Part model, mm, in its own coordinate system. Face numbers are marked on the shaded views. A direction names the side the tool comes from. Coordinates: 2 decimals unless noted, no trailing zeros. Loops run counter-clockwise (first coordinate to the right, second up) from the corner with the lowest first, then second, coordinate; pieces in that order, holes last. Notation, with made-up numbers: (65, 5.25) -> (110, 5.25) arc R26 ccw to (110, 38.25) -> close; hole circle Ø11 at (86.5, 69). An arc over 180 degrees is marked (long way). Use one line per item in the form item = value. Start each with the question number.
(1) 3-axis set-ups, long thin cutter, end or side, ignore diameter. For the marked faces 1 and 2: which of +Z, -Z, +X, -X, +Y, -Y reach the whole face in a straight line?
(2) Band-saw the part on D-D on x = -31. Give the cut face in (y, z), then the cut area to 3 significant figures.
(3) Band-saw the part on B-B on x = 0. Give the cut face in (y, z), then the cut area to 3 significant figures.
(4) Pin check, flat tips, straight feed: P1, Ø6, axis at x = 22, y = 15, coming from the -Z side; P2, Ø1.5, axis at x = 22.5, y = 5.5, coming from the -Z side; P3, Ø2, axis at x = -4, y = 7, coming from the -Z side. Stop position of each tip, or through.
(5) Mould opens along X. For the marked faces 3, 4 and 5 say: +X half, -X half, draft (parallel to the pull), parting line (faces both ways), or undercut.
(6) Band-saw the part on C-C on y = 31.5. Give the cut face in (x, z), then the cut area to 3 significant figures.
(7) Drill centre lines: L1, parallel to X at y = 10, z = 0; L2, parallel to X at y = 24, z = 0; L3, parallel to Y at x = -5, z = -23. Where is each one in solid material? Low to high. Write a range as [from, to].
(8) Band-saw the part on A-A on z = 0. Give the cut face in (x, y), then the cut area to 3 significant figures.
```python
from build123d import *

# Parameters (mm, degrees)
SKETCH1_R          = 38.1
EXTRUDE1_DEPTH     = 12.7
SKETCH2_R          = 19.05
EXTRUDE2_DEPTH     = 25.4
SKETCH3_R          = 12.7
CUT_EXTRUDE1_DEPTH = 66.991135768


with BuildPart() as part:
    # Sketch1 → Extrude1 (new body)
    with BuildSketch(Plane(origin=(0, 0, 0), x_dir=(1, 0, 0), z_dir=(0, 1, 0))):
        with Locations(Location((0, 0, 0), (0, 0, 270))):
            Circle(SKETCH1_R)
    extrude(amount=EXTRUDE1_DEPTH)

    # Sketch2 → Extrude2 (add)
    with BuildSketch(Plane(origin=(0, 12.7, 0), x_dir=(-1, 0, 0), z_dir=(0, 1, 0))):
        with Locations(Location((0, 0, 0), (0, 0, 90))):
            Circle(SKETCH2_R)
    extrude(amount=EXTRUDE2_DEPTH)

    # Sketch3 → Cut-Extrude1 (cut, through all)
    with BuildSketch(Plane(origin=(0, 38.1, 0), x_dir=(-1, 0, 0), z_dir=(0, 1, 0))):
        with Locations(Location((0, 0, 0), (0, 0, 90))):
            Circle(SKETCH3_R)
    extrude(amount=-CUT_EXTRUDE1_DEPTH, mode=Mode.SUBTRACT)


solid = part.part
```
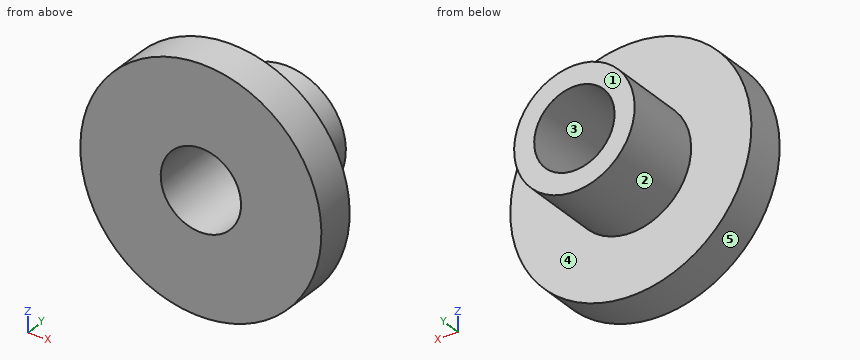
A:
q1.face_1 = +Z, -Z, +X, -X, +Y
q1.face_2 = +Y
q2.outline = (0, -22.15) -> (12.7, -22.15) -> (12.7, 22.15) -> (0, 22.15) -> close
q2.area = 563 mm²
q3.outline = (0, -38.1) -> (12.7, -38.1) -> (12.7, -19.05) -> (38.1, -19.05) -> (38.1, -12.7) -> (0, -12.7) -> close; (0, 12.7) -> (38.1, 12.7) -> (38.1, 19.05) -> (12.7, 19.05) -> (12.7, 38.1) -> (0, 38.1) -> close
q3.area = 968 mm²
q4.P1 = -32.38
q4.P2 = -31.28
q4.P3 = -37.98
q5.face_3 = undercut
q5.face_4 = draft
q5.face_5 = parting line
q6.outline = circle Ø38.1 at (0, 0); hole circle Ø25.4 at (0, 0)
q6.area = 633 mm²
q7.L1 = [-38.1, -12.7], [12.7, 38.1]
q7.L2 = [-19.05, -12.7], [12.7, 19.05]
q7.L3 = [0, 12.7]
q8.outline = (-38.1, 0) -> (-12.7, 0) -> (-12.7, 38.1) -> (-19.05, 38.1) -> (-19.05, 12.7) -> (-38.1, 12.7) -> close; (12.7, 0) -> (38.1, 0) -> (38.1, 12.7) -> (19.05, 12.7) -> (19.05, 38.1) -> (12.7, 38.1) -> close
q8.area = 968 mm²
